```python
from build123d import *

# Parameters (mm, degrees)
SKETCH1_W                     = 935.7
SKETCH1_H                     = 528
BASE_FLANGE1_DEPTH            = 1.7366
EDGE_FLANGE1_STRIP_W          = 8.4196
EDGE_FLANGE1_STRIP_H          = 1.7366
EDGE_FLANGE1_STRIP_CUT_DEPTH  = 931.7
EDGE_FLANGE1_RELIEF_W         = 9.2879
EDGE_FLANGE1_RELIEF_H         = 0.8683
EDGE_FLANGE1_RELIEF_CUT_DEPTH = 1.7366
EDGE_FLANGE1_DEPTH            = 931.7
EDGE_FLANGE2_STRIP_W          = 8.4196
EDGE_FLANGE2_STRIP_H          = 1.7366
EDGE_FLANGE2_STRIP_CUT_DEPTH  = 931.7
EDGE_FLANGE2_RELIEF_W         = 9.2879
EDGE_FLANGE2_RELIEF_H         = 0.8683
EDGE_FLANGE2_RELIEF_CUT_DEPTH = 1.7366
EDGE_FLANGE2_DEPTH            = 931.7
EDGE_FLANGE4_STRIP_W          = 8.4196
EDGE_FLANGE4_STRIP_H          = 1.7366
EDGE_FLANGE4_STRIP_CUT_DEPTH  = 528
EDGE_FLANGE4_DEPTH            = 528
EDGE_FLANGE5_STRIP_W          = 8.4196
EDGE_FLANGE5_STRIP_H          = 1.7366
EDGE_FLANGE5_STRIP_CUT_DEPTH  = 528
EDGE_FLANGE5_DEPTH            = 528


# Sheet-metal steps are written as plain solids
with BuildPart() as part:
    # Sketch1 → Base-Flange1 (new body)
    with BuildSketch(Plane(origin=(0, 0, 0), x_dir=(0, 0, -1), z_dir=(1, 0, 0))):
        Rectangle(SKETCH1_W, SKETCH1_H)
    extrude(amount=-BASE_FLANGE1_DEPTH)

    # Edge-Flange1 strip (across the edge) → Edge-Flange1 strip cut (cut)
    with BuildSketch(Plane(origin=(0, 264, -465.85), x_dir=(0, -1, 0), z_dir=(0, 0, 1))):
        with Locations((-1.7366, -0.8683)):
            Rectangle(EDGE_FLANGE1_STRIP_W, EDGE_FLANGE1_STRIP_H)
    extrude(amount=EDGE_FLANGE1_STRIP_CUT_DEPTH, mode=Mode.SUBTRACT)

    # Edge-Flange1 relief (on the sheet) → Edge-Flange1 relief cut (cut)
    with BuildSketch(Plane(origin=(0, 261.5268, -465.85), x_dir=(0, -1, 0), z_dir=(1, 0, 0))):
        with Locations((-3.77565, 0.43415)):
            Rectangle(EDGE_FLANGE1_RELIEF_W, EDGE_FLANGE1_RELIEF_H)
        with Locations((-3.77565, -932.13415)):
            Rectangle(EDGE_FLANGE1_RELIEF_W, EDGE_FLANGE1_RELIEF_H)
    extrude(amount=-EDGE_FLANGE1_RELIEF_CUT_DEPTH, mode=Mode.SUBTRACT)

    # Edge-Flange1 section (across the edge) → Edge-Flange1 (add)
    with BuildSketch(Plane(origin=(0, 264, -465.85), x_dir=(0, -1, 0), z_dir=(0, 0, 1))):
        with BuildLine():
            Line((0, 0.7366), (0, 28.2634))
            Line((0, 28.2634), (1.7366, 28.2634))
            Line((1.7366, 28.2634), (1.7366, 0.7366))
            ThreePointArc((1.7366, 0.7366), (1.952345145, 0.215745145), (2.4732, 0))
            Line((2.4732, 0), (2.4732, -1.7366))
            ThreePointArc((2.4732, -1.7366), (0.724383509, -1.012216491), (0, 0.7366))
        make_face()
    extrude(amount=EDGE_FLANGE1_DEPTH)

    # Edge-Flange2 strip (across the edge) → Edge-Flange2 strip cut (cut)
    with BuildSketch(Plane(origin=(0, -264, 465.85), x_dir=(0, 1, 0), z_dir=(0, 0, -1))):
        with Locations((-1.7366, -0.8683)):
            Rectangle(EDGE_FLANGE2_STRIP_W, EDGE_FLANGE2_STRIP_H)
    extrude(amount=EDGE_FLANGE2_STRIP_CUT_DEPTH, mode=Mode.SUBTRACT)

    # Edge-Flange2 relief (on the sheet) → Edge-Flange2 relief cut (cut)
    with BuildSketch(Plane(origin=(0, -261.5268, 465.85), x_dir=(0, 1, 0), z_dir=(1, 0, 0))):
        with Locations((-3.77565, 0.43415)):
            Rectangle(EDGE_FLANGE2_RELIEF_W, EDGE_FLANGE2_RELIEF_H)
        with Locations((-3.77565, -932.13415)):
            Rectangle(EDGE_FLANGE2_RELIEF_W, EDGE_FLANGE2_RELIEF_H)
    extrude(amount=-EDGE_FLANGE2_RELIEF_CUT_DEPTH, mode=Mode.SUBTRACT)

    # Edge-Flange2 section (across the edge) → Edge-Flange2 (add)
    with BuildSketch(Plane(origin=(0, -264, 465.85), x_dir=(0, 1, 0), z_dir=(0, 0, -1))):
        with BuildLine():
            Line((0, 0.7366), (0, 28.2634))
            Line((0, 28.2634), (1.7366, 28.2634))
            Line((1.7366, 28.2634), (1.7366, 0.7366))
            ThreePointArc((1.7366, 0.7366), (1.952345145, 0.215745145), (2.4732, 0))
            Line((2.4732, 0), (2.4732, -1.7366))
            ThreePointArc((2.4732, -1.7366), (0.724383509, -1.012216491), (0, 0.7366))
        make_face()
    extrude(amount=EDGE_FLANGE2_DEPTH)

    # Edge-Flange4 strip (across the edge) → Edge-Flange4 strip cut (cut)
    with BuildSketch(Plane(origin=(0, 264, 467.85), x_dir=(0, 0, -1), z_dir=(0, -1, 0))):
        with Locations((-3.4732, -0.8683)):
            Rectangle(EDGE_FLANGE4_STRIP_W, EDGE_FLANGE4_STRIP_H)
    extrude(amount=EDGE_FLANGE4_STRIP_CUT_DEPTH, mode=Mode.SUBTRACT)

    # Edge-Flange4 section (across the edge) → Edge-Flange4 (add)
    with BuildSketch(Plane(origin=(0, 264, 467.85), x_dir=(0, 0, -1), z_dir=(0, -1, 0))):
        with BuildLine():
            Line((-1.7366, 0.7366), (-1.7366, 28.2634))
            Line((-1.7366, 28.2634), (0, 28.2634))
            Line((0, 28.2634), (0, 0.7366))
            ThreePointArc((0, 0.7366), (0.215745145, 0.215745145), (0.7366, 0))
            Line((0.7366, 0), (0.7366, -1.7366))
            ThreePointArc((0.7366, -1.7366), (-1.012216491, -1.012216491), (-1.7366, 0.7366))
        make_face()
    extrude(amount=EDGE_FLANGE4_DEPTH)

    # Edge-Flange5 strip (across the edge) → Edge-Flange5 strip cut (cut)
    with BuildSketch(Plane(origin=(0, -264, -467.85), x_dir=(0, 0, 1), z_dir=(0, 1, 0))):
        with Locations((-3.4732, -0.8683)):
            Rectangle(EDGE_FLANGE5_STRIP_W, EDGE_FLANGE5_STRIP_H)
    extrude(amount=EDGE_FLANGE5_STRIP_CUT_DEPTH, mode=Mode.SUBTRACT)

    # Edge-Flange5 section (across the edge) → Edge-Flange5 (add)
    with BuildSketch(Plane(origin=(0, -264, -467.85), x_dir=(0, 0, 1), z_dir=(0, 1, 0))):
        with BuildLine():
            Line((-1.7366, 0.7366), (-1.7366, 28.2634))
            Line((-1.7366, 28.2634), (0, 28.2634))
            Line((0, 28.2634), (0, 0.7366))
            ThreePointArc((0, 0.7366), (0.215745145, 0.215745145), (0.7366, 0))
            Line((0.7366, 0), (0.7366, -1.7366))
            ThreePointArc((0.7366, -1.7366), (-1.012216491, -1.012216491), (-1.7366, 0.7366))
        make_face()
    extrude(amount=EDGE_FLANGE5_DEPTH)


solid = part.part
```
Geometry check sheet. Reference: the model listing, model coordinates, mm. A direction names the side the tool comes from. Round coordinates to 2 decimals unless told otherwise and drop trailing zeros. Order: outer loops, then holes, each group sorted by start corner. A loop starts at its lowest first (then second) coordinate and runs counter-clockwise, first axis right, second up. Notation, with made-up numbers: (-17.75, -22.75) - (35.25, -22.75) arc R34 cw to (35.25, 8.25) - close; hole circle Ø8 at (44, -11). An arc over 180 degrees is marked (long way). Use a Markdown table: item, result. Add a question column.
(1) Depth check by flat-ended pin: pin 1 (4 mm diameter, centred on y = 170, z = -139, fed in from +X); pin 2 (1.9 mm diameter, centred on x = -1, y = 262.5, fed in from +Z); pin 3 (0.7 mm diameter, centred on x = -1, z = -466, fed in from +Y). Enter the tip coordinate at first touch or a pass-through.
(2) Tool access check on faces 4 (the flat face through (15, -262.263, 7)), 5 (the flat face through (15, 4, 467.85)), 6 (the flat face through (14, 4, 469.587)). Record the directions out of +Z, -Z, +X, -X, +Y, -Y that give a thin tool (end or side, any length) a straight path to the whole face; none if there is none.
(3) Sectioned sample at A-A, the plane x = 12.5. Enter the section's corners in (y, z).
(4) Release check for a two-part mould opening along Y. For faces 1 (the flat face through (14, -264, 7)), 2 (the flat face through (15, 262.263, -7)), 3 (the flat face through (-1.737, 4, 7)) record: pulls with the +Y half, pulls with the -Y half, needs draft (parallel to the pull), parting line crosses it, or undercut.
(5) Sectioned sample at C-C, the plane y = -148. Enter the section's corners in (x, z).
(6) Material ranges on line 1 along Z through (x, y) = (3, -77); line 2 along Y through (x, z) = (10.25, 99); line 3 along X through (y, z) = (204.5, -400), recorded low to high. Write a range as [from, to].
(7) Sectioned sample at B-B, the plane z = 263. Enter the section's corners in (x, y), and give its area (3 significant figures).
Answers below:
| question | item | result |
|---|---|---|
| 1 | pin 1 | x = 0 |
| 1 | pin 2 | z = 469.46 |
| 1 | pin 3 | y = 263.55 |
| 2 | face 4 | +X |
| 2 | face 5 | +X, +Y, -Y |
| 2 | face 6 | +Z, +X, -X, +Y, -Y |
| 3 | outline | (-264, -469.59) - (264, -469.59) - (264, -467.85) - (-264, -467.85) - close; (-264, -465.85) - (-262.26, -465.85) - (-262.26, 465.85) - (-264, 465.85) - close; (-264, 467.85) - (264, 467.85) - (264, 469.59) - (-264, 469.59) - close; (262.26, -465.85) - (264, -465.85) - (264, 465.85) - (262.26, 465.85) - close |
| 4 | face 1 | pulls with the -Y half |
| 4 | face 2 | undercut |
| 4 | face 3 | needs draft |
| 5 | outline | (-1.74, -467.11) arc R2.47 ccw to (0.74, -469.59) - (28.26, -469.59) - (28.26, -467.85) - (0.74, -467.85) arc R0.74 cw to (0, -467.11) - (0, 467.11) arc R0.74 cw to (0.74, 467.85) - (28.26, 467.85) - (28.26, 469.59) - (0.74, 469.59) arc R2.47 ccw to (-1.74, 467.11) - close |
| 6 | line 1 | [-469.59, -467.85], [467.85, 469.59] |
| 6 | line 2 | [-264, -262.26], [262.26, 264] |
| 6 | line 3 | [-1.74, 0] |
| 7 | outline | (-1.74, -261.53) arc R2.47 ccw to (0.74, -264) - (28.26, -264) - (28.26, -262.26) - (0.74, -262.26) arc R0.74 cw to (0, -261.53) - (0, 261.53) arc R0.74 cw to (0.74, 262.26) - (28.26, 262.26) - (28.26, 264) - (0.74, 264) arc R2.47 ccw to (-1.74, 261.53) - close |
| 7 | area | 1,010 mm² |
